Design review of the part built by this model. Coordinates are the model's own, in mm. Face numbers are marked on the shaded views. Give positions to 0.01 mm unless a question says otherwise; leave off trailing zeros. Write each loop counter-clockwise with the first axis right and the second up, starting at its lowest first coordinate (ties: lowest second). Pieces come first, ordered by that corner, then holes. Notation, with made-up numbers: M 86,-36.75 L 127,-36.75 A31 ccw 127,-3.75 Z; hole C 4.25,-39 d6. An arc over 180 degrees is marked long. Answer in a Markdown table with one row per item.
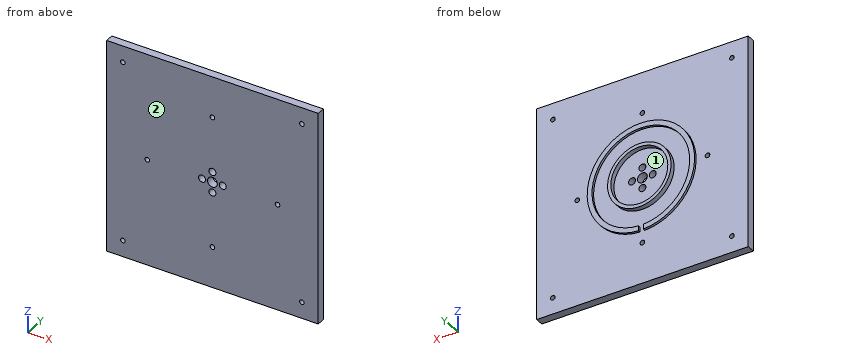
```python
from build123d import *

# Parameters (mm, degrees)
SKETCH1_W           = 130
SKETCH1_H           = 130
SKETCH1_R           = 31
SKETCH1_R_2         = 26
SKETCH1_R_3         = 24
BOSS_EXTRUDE2_DEPTH = 5
SKETCH2_R           = 33
SKETCH2_R_2         = 30
BOSS_EXTRUDE3_DEPTH = 1.5
SKETCH3_R           = 2.15
SKETCH3_R_2         = 3
CUT_EXTRUDE1_DEPTH  = 5
SKETCH5_R           = 1.42
CUT_EXTRUDE3_DEPTH  = 10
SKETCH6_R           = 19.5
SKETCH6_R_2         = 17.5
BOSS_EXTRUDE4_DEPTH = 3
SKETCH7_W           = 3
SKETCH7_H           = 7.819809603
CUT_EXTRUDE5_DEPTH  = 1.5


with BuildPart() as part:
    # Sketch1 → Boss-Extrude2 (new body)
    # profile 1 of 4: a face of its own
    with BuildSketch(Plane(origin=(0, 0, 0), x_dir=(1, 0, 0), z_dir=(0, 1, 0))):
        Rectangle(SKETCH1_W, SKETCH1_H)
        Circle(SKETCH1_R, mode=Mode.SUBTRACT)
    # profile 2 of 4: a face of its own
    with BuildSketch(Plane(origin=(0, 0, 0), x_dir=(1, 0, 0), z_dir=(0, 1, 0))):
        Circle(SKETCH1_R)
        Circle(SKETCH1_R_2, mode=Mode.SUBTRACT)
    # profile 3 of 4: a face of its own
    with BuildSketch(Plane(origin=(0, 0, 0), x_dir=(1, 0, 0), z_dir=(0, 1, 0))):
        Circle(SKETCH1_R_2)
        Circle(SKETCH1_R_3, mode=Mode.SUBTRACT)
    # profile 4 of 4: a face of its own
    with BuildSketch(Plane(origin=(0, 0, 0), x_dir=(1, 0, 0), z_dir=(0, 1, 0))):
        Circle(SKETCH1_R_3)
    extrude(amount=BOSS_EXTRUDE2_DEPTH)

    # Sketch2 → Boss-Extrude3 (add)
    with BuildSketch(Plane(origin=(0, 5, 0), x_dir=(1, 0, 0), z_dir=(0, 1, 0))):
        with Locations(Location((0, 0, 0), (0, 0, 270))):
            Circle(SKETCH2_R)
        with Locations(Location((0, 0, 0), (0, 0, 270))):
            Circle(SKETCH2_R_2, mode=Mode.SUBTRACT)
    extrude(amount=BOSS_EXTRUDE3_DEPTH)

    # Sketch3 → Cut-Extrude1 (cut)
    with BuildSketch(Plane(origin=(0, 5, 0), x_dir=(1, 0, 0), z_dir=(0, 1, 0))):
        with Locations(Location((0, 6.35, 0), (0, 0, 270))):
            Circle(SKETCH3_R)
        with Locations(Location((6.35, 0, 0), (0, 0, 270))):
            Circle(SKETCH3_R)
        with Locations(Location((0, -6.35, 0), (0, 0, 270))):
            Circle(SKETCH3_R)
        with Locations(Location((-6.35, 0, 0), (0, 0, 270))):
            Circle(SKETCH3_R)
        with Locations(Location((0, 0, 0), (0, 0, 270))):
            Circle(SKETCH3_R_2)
    extrude(amount=-CUT_EXTRUDE1_DEPTH, mode=Mode.SUBTRACT)

    # Sketch5 → Cut-Extrude3 (cut)
    with BuildSketch(Plane(origin=(0, 5, 0), x_dir=(1, 0, 0), z_dir=(0, 1, 0))):
        with Locations(Location((-55, 55, 0), (0, 0, 270))):
            Circle(SKETCH5_R)
        with Locations(Location((-55, -55, 0), (0, 0, 270))):
            Circle(SKETCH5_R)
        with Locations(Location((55, -55, 0), (0, 0, 270))):
            Circle(SKETCH5_R)
        with Locations(Location((55, 55, 0), (0, 0, 270))):
            Circle(SKETCH5_R)
        with Locations(Location((0, 40, 0), (0, 0, 270))):
            Circle(SKETCH5_R)
        with Locations(Location((-40, 0, 0), (0, 0, 270))):
            Circle(SKETCH5_R)
        with Locations(Location((40, 0, 0), (0, 0, 270))):
            Circle(SKETCH5_R)
        with Locations(Location((0, -40, 0), (0, 0, 270))):
            Circle(SKETCH5_R)
    extrude(amount=-CUT_EXTRUDE3_DEPTH, mode=Mode.SUBTRACT)

    # Sketch6 → Boss-Extrude4 (add)
    with BuildSketch(Plane(origin=(0, 5, 0), x_dir=(1, 0, 0), z_dir=(0, 1, 0))):
        with Locations(Location((0, 0, 0), (0, 0, 270))):
            Circle(SKETCH6_R)
        with Locations(Location((0, 0, 0), (0, 0, 270))):
            Circle(SKETCH6_R_2, mode=Mode.SUBTRACT)
    extrude(amount=BOSS_EXTRUDE4_DEPTH)

    # Sketch7 → Cut-Extrude5 (cut)
    with BuildSketch(Plane(origin=(0, 6.5, 0), x_dir=(1, 0, 0), z_dir=(0, 1, 0))):
        with Locations((0, 31.405364374)):
            Rectangle(SKETCH7_W, SKETCH7_H)
    extrude(amount=-CUT_EXTRUDE5_DEPTH, mode=Mode.SUBTRACT)


solid = part.part
```
1) Add section C-C (x = -13). Write out the cut boundary in (y, z), and give its area (3 significant figures).
Geometry says:
| item | result |
|---|---|
| outline | M 0,-65 L 5,-65 L 5,-30.33 L 6.5,-30.33 L 6.5,-27.04 L 5,-27.04 L 5,-14.53 L 8,-14.53 L 8,-11.72 L 5,-11.72 L 5,11.72 L 8,11.72 L 8,14.53 L 5,14.53 L 5,27.04 L 6.5,27.04 L 6.5,30.33 L 5,30.33 L 5,65 L 0,65 Z |
| area | 677 mm^2 |
2) To check wall thickness, follow probe 1 along X at (y, z) = (1.45, 0); probe 2 along X at (y, z) = (3.2, 55); probe 3 along X at (y, z) = (2.1, -6.35). State the ranges of each line that lie inside material, in increasing order. Write a range as [from, to].
Geometry says:
| item | result |
|---|---|
| probe 1 | [-65, -41.42], [-38.58, -8.5], [-4.2, -3], [3, 4.2], [8.5, 38.58], [41.42, 65] |
| probe 2 | [-65, -56.42], [-53.58, 53.58], [56.42, 65] |
| probe 3 | [-65, -2.15], [2.15, 65] |
3) Add section A-A (x = 6.35). Write out the cut boundary in (y, z), and give its area (3 significant figures).
Geometry says:
| item | result |
|---|---|
| outline | M 0,-65 L 5,-65 L 5,-32.38 L 6.5,-32.38 L 6.5,-29.32 L 5,-29.32 L 5,-18.44 L 8,-18.44 L 8,-16.31 L 5,-16.31 L 5,-2.15 L 0,-2.15 Z; M 0,2.15 L 5,2.15 L 5,16.31 L 8,16.31 L 8,18.44 L 5,18.44 L 5,29.32 L 6.5,29.32 L 6.5,32.38 L 5,32.38 L 5,65 L 0,65 Z |
| area | 650 mm^2 |
4) Insertion check: P1, Ø1.2, axis at y = 5.5, z = -31, coming from the -X side; P2, Ø9.5, axis at x = 0, z = 0, coming from the +Y side; P3, Ø8, axis at x = -2, z = -29.5, coming from the +Y side. Each pin has a flat end and moves straight along its axis. Give the tip position at first contact, or say it passes through.
Geometry says:
| item | result |
|---|---|
| P1 | x = -65 |
| P2 | y = 5 |
| P3 | y = 6.5 |
5) The part is to be moulded in two halves that separate along Z. For the marked faces 1 and 2, say which applies: released by +Z, released by -Z, zero draft, split by the parting line, or undercut.
Geometry says:
| item | result |
|---|---|
| face 1 | undercut |
| face 2 | zero draft |
6) Add section D-D (z = 26.5). Write out the cut boundary in (x, y).
Geometry says:
| item | result |
|---|---|
| outline | M -65,0 L 65,0 L 65,5 L 19.67,5 L 19.67,6.5 L 14.06,6.5 L 14.06,5 L -14.06,5 L -14.06,6.5 L -19.67,6.5 L -19.67,5 L -65,5 Z |
7) Add section B-B (z = -6.35). Write out the cut boundary in (x, y), and give its area (3 significant figures).
Geometry says:
| item | result |
|---|---|
| outline | M -65,0 L -2.15,0 L -2.15,5 L -16.31,5 L -16.31,8 L -18.44,8 L -18.44,5 L -29.32,5 L -29.32,6.5 L -32.38,6.5 L -32.38,5 L -65,5 Z; M 2.15,0 L 65,0 L 65,5 L 32.38,5 L 32.38,6.5 L 29.32,6.5 L 29.32,5 L 18.44,5 L 18.44,8 L 16.31,8 L 16.31,5 L 2.15,5 Z |
| area | 650 mm^2 |
